The drawing under review shows one solid part. Ordinate dimensions are in mm from its lowest x, y, z. A direction names the side the tool comes from. Coordinates: 2 decimals unless noted, no trailing zeros. Loops run counter-clockwise (first coordinate to the right, second up) from the corner with the lowest first, then second, coordinate; pieces in that order, holes last. Notation, with made-up numbers: (61.5, 26) -> (73.5, 26) arc R20 ccw to (73.5, 40) -> close; hole circle Ø8 at (64.5, -10.5). An arc over 180 degrees is marked (long way). Use a Markdown table: item, result.
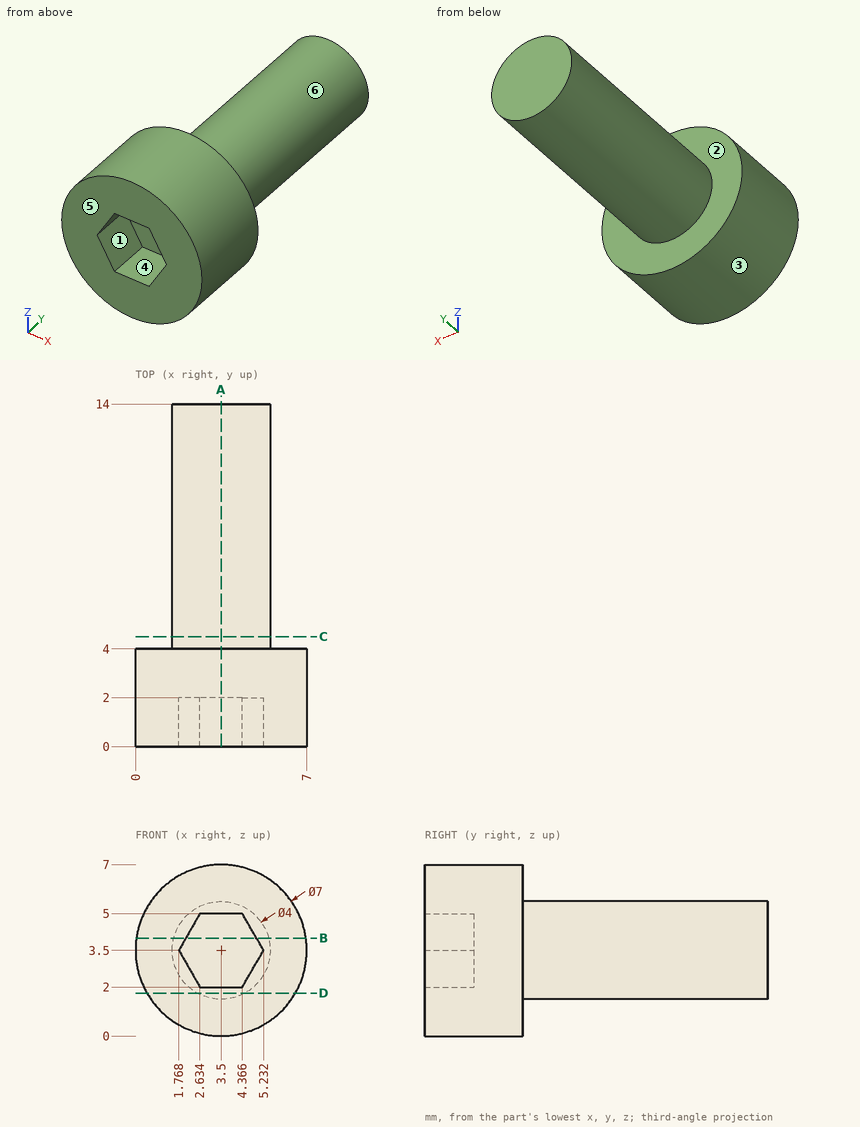
(1) For the marked faces 1, 2 and 3, list the 3-axis set-ups (+Z, -Z, +X, -X, +Y, -Y) from which the entire face can be reached by the end or side of a thin tool; tool diameter is ignored.
Found:
| item | result |
|---|---|
| face 1 | -Y |
| face 2 | +Y |
| face 3 | +Y, -Y |
(2) For line 1 along Y through (x, z) = (4, 2.25); line 2 along Y through (x, z) = (0.5, 4.25); line 3 along Z through (x, y) = (2.5, 10.25), list the stretches that pass through material, from the lowest coordinate up.
Found:
| item | result |
|---|---|
| line 1 | y = 2 to 14 |
| line 2 | y = 0 to 4 |
| line 3 | z = 1.77 to 5.23 |
(3) For pin 1 Ø1 at (y, z) = (7.5, 4) entering from -X; pin 2 Ø1.5 at (x, z) = (3, 3) entering from -Y, all flat-tipped, find the tip position at first contact; note any pin that passes through.
Found:
| item | result |
|---|---|
| pin 1 | stops at x = 1.5 |
| pin 2 | stops at y = 2 |
(4) Take a section at B-B on z = 4. Write out the cut boundary in (x, y).
Found:
| item | result |
|---|---|
| outline | (0.04, 0) -> (2.06, 0) -> (2.06, 2) -> (4.94, 2) -> (4.94, 0) -> (6.96, 0) -> (6.96, 4) -> (5.44, 4) -> (5.44, 14) -> (1.56, 14) -> (1.56, 4) -> (0.04, 4) -> close |
(5) Take a section at A-A on x = 3.5. Write out the cut boundary in (y, z), plus the area to 3 significant figures.
Found:
| item | result |
|---|---|
| outline | (0, 0) -> (4, 0) -> (4, 1.5) -> (14, 1.5) -> (14, 5.5) -> (4, 5.5) -> (4, 7) -> (0, 7) -> (0, 5) -> (2, 5) -> (2, 2) -> (0, 2) -> close |
| area | 62.0 mm^2 |
(6) Mouldability with a two-part tool opening along Z and no side actions: class the marked faces 4, 5 and 6 as pulls with the +Z half, pulls with the -Z half, needs draft (parallel to the pull), parting line crosses it, or undercut.
Found:
| item | result |
|---|---|
| face 4 | undercut |
| face 5 | needs draft |
| face 6 | parting line crosses it |
(7) Take a section at C-C on y = 4.5. Write out the cut boundary in (x, z), plus the area to 3 significant figures.
Found:
| item | result |
|---|---|
| outline | circle Ø4 at (3.5, 3.5) |
| area | 12.6 mm^2 |
(8) Take a section at D-D on z = 1.75. Write out the cut boundary in (x, y).
Found:
| item | result |
|---|---|
| outline | (0.47, 0) -> (6.53, 0) -> (6.53, 4) -> (4.47, 4) -> (4.47, 14) -> (2.53, 14) -> (2.53, 4) -> (0.47, 4) -> close |
